The listing builds one solid part. Answer for the finished solid, in the listing's coordinates (mm). A direction names the side the tool comes from. Coordinates: 2 decimals unless noted, no trailing zeros. Order: outer loops, then holes, each group sorted by start corner. A loop starts at its lowest first (then second) coordinate and runs counter-clockwise, first axis right, second up. Notation, with made-up numbers: (-37, 49.25) - (-31, 49.25) arc R27 cw to (-31, 80.25) - close; hole circle Ø11 at (-28, 85.5). An arc over 180 degrees is marked (long way). Use one line per item in the form item = value. Start each with the question number.
Item 1: A tool of negligible diameter and unlimited length cuts with its end or side. For faces 1 (the flat face through (70, -93, -3)), 2 (the flat face through (78, -88, -4)), 3 (the flat face through (65.5, -96, -4)), from which of +Z, -Z, +X, -X, +Y, -Y can it reach the whole face along a straight path? Write none if from no direction.
Item 2: The mould has two halves that part along Y. Classify faces 4 (the flat face through (40, 2, 1)), 5 (the flat face through (78, -43, -4)), 6 (the flat face through (80.5, -58.4, 0.4)): released by +Y, released by -Y, zero draft, split by the parting line, or undercut.
Item 3: Consider line 1 along Y through (x, z) = (78.4, -4); line 2 along Z through (x, y) = (78, -38); line 3 along Y through (x, z) = (27, 1). Determine where each line is inside the solid, lowest interval first. Write a range as [from, to].
Item 4: Section C-C, the plane x = 19.5 is taken. Write down the section's boundary in (y, z).
Item 5: Section B-B, the plane y = -48 is taken. Write down the section's boundary in (x, z), and give its area (3 significant figures).
Item 6: Each of these flat-tipped pins is pushed along its axis until it touches: pin 1 Ø1 at (x, z) = (42.5, -6.5) entering from +Y; pin 2 Ø4 at (y, z) = (-90, -4) entering from -X; pin 3 Ø4 at (x, z) = (77, -5) entering from +Y; pin 4 Ø1.2 at (x, z) = (70.5, -4) entering from -Y. Where does it stop, or does it pass through?
Item 7: Section A-A, the plane y = -4 is taken. Write down the section's boundary in (x, z), and give its area (3 significant figures).
Item 8: Section D-D, the plane y = -18 is taken. Write down the section's boundary in (x, z), and give its area (3 significant figures).
Autodesk Inventor part; units mm, degrees
ref_plane "YZ Plane" through (0, 0, 0) normal (1, 0, 0) x (0, 1, 0)
ref_plane "XZ Plane" through (0, 0, 0) normal (0, 1, 0) x (-1, 0, 0)
ref_plane "XY Plane" through (0, 0, 0) normal (0, 0, 1) x (1, 0, 0)
ref_plane "Work Plane1" through (0, 0, 0) normal (0, 0, 1) x (1, 0, 0)
sketch "Sketch1" plane through (0, 0, 0) normal (0, 0, 1) x (1, 0, 0)
  line L0 (-2, -98) -> (8, -98)
  line L1 (-2, -98) -> (-2, 2)
  circle A0 centre (4, -93) radius 0.75
  circle A1 centre (4, -48) radius 0.75
  circle A2 centre (5, -4) radius 0.75
  line L2 (0, 2) -> (80.5, 2)
  circle A3 centre (40.25, -4) radius 0.75
  circle A4 centre (75.5, -4) radius 0.75
  line L3 (34.223, -24.7194) -> (34.223, -14.2194)
  line L4 (26.723, -24.7194) -> (34.223, -24.7194)
  line L5 (26.723, -14.2194) -> (26.723, -24.7194)
  line L6 (34.223, -14.2194) -> (26.723, -14.2194)
  line L7 (80.5, 2) -> (-2, 2)
  line L8 (-2, 2) -> (-2, -98)
  line L9 (-2, -98) -> (80.5, -98)
  line L10 (80.5, -98) -> (80.5, 2)
  point P0 (0, 0)
  point P1 (20.6901, -14.1894)
extrude "Extrusion1" add sketch "Sketch1" along normal blind 2
sketch "Sketch2" plane through (0, 0, 0) normal (0, 0, -1) x (-1, 0, 0)
  point P0 (0, 0)
sketch "Sketch3" plane through (0, 0, 0) normal (0, 0, -1) x (-1, 0, 0)
  point P0 (0, 0)
sketch "Sketch4" plane through (80.5, -98, 0) normal (1, 0, 0) x (0, 0, -1)
  line L0 (0, 45) -> (0, 55)
  line L1 (0, 45) -> (5, 45)
  line L2 (5, 55) -> (5, 45)
  line L3 (0, 55) -> (5, 55)
  line L4 (0, 45) -> (8, 45)
  line L5 (8, 45) -> (8, 55)
  line L6 (8, 55) -> (0, 55)
  circle A0 centre (4, 50) radius 0.75
  point P0 (0, 98)
  dimension "d3" = 8
  dimension "d4" = 10
  dimension "d6" = 1.5
extrude "Extrusion2" add sketch "Sketch4" against normal blind 5
sketch "Sketch5" plane through (80.5, -98, 2) normal (1, 0, 0) x (0, 0, -1)
  line L0 (2, 45) -> (2, 0)
  line L1 (2, 0) -> (10, 0)
  line L2 (10, 0) -> (10, 10)
  line L3 (10, 10) -> (2, 10)
  line L4 (2, 10) -> (2, 0)
  circle A0 centre (6, 5) radius 0.75
  point P0 (2, 98)
  dimension "d9" = 8
  dimension "d10" = 10
  dimension "d12" = 1.5
extrude "Extrusion3" add sketch "Sketch5" against normal blind 5
sketch "Sketch6" plane through (-2, -98, 2) normal (0, -1, 0) x (1, 0, 0)
  line L0 (77.5, -10) -> (77.5, -2)
  line L1 (77.5, -10) -> (67.5, -10)
  line L2 (67.5, -10) -> (67.5, -2)
  line L3 (67.5, -2) -> (77.5, -2)
  line L4 (77.5, -2) -> (77.5, -10)
  circle A0 centre (72.5, -6) radius 0.75
  point P0 (2, -2)
  dimension "d15" = 10
  dimension "d16" = 8
  dimension "d18" = 1.5
extrude "Extrusion4" add sketch "Sketch6" against normal blind 5
sketch "Sketch7" plane through (-2, -98, 2) normal (0, -1, 0) x (1, 0, 0)
  line L0 (10, -2) -> (10, -17)
  line L1 (67.5, -10) -> (67.5, -2)
  circle A0 centre (32.473, -6) radius 0.75
  line L2 (32.473, -10) -> (27.473, -10)
  line L3 (27.473, -10) -> (27.473, -2)
  line L4 (27.473, -2) -> (37.473, -2)
  line L5 (37.473, -2) -> (37.473, -10)
  line L6 (37.473, -10) -> (32.473, -10)
  point P0 (2, -2)
  dimension "d22" = 1.5
  dimension "d25" = 4
  dimension "d26" = 5
  dimension "d27" = 8
  dimension "d28" = 10
  dimension "d29" = 8
extrude "Extrusion5" add sketch "Sketch7" against normal blind 5
sketch "Sketch8" plane through (-2, -98, 2) normal (0, -1, 0) x (1, 0, 0)
  line L0 (37.473, -10) -> (27.473, -10)
  line L1 (27.473, -10) -> (37.473, -10)
  line L2 (37.473, -10) -> (37.473, -2)
  line L3 (37.473, -2) -> (27.473, -2)
  line L4 (27.473, -2) -> (27.473, -10)
  point P0 (2, -2)
extrude "Extrusion6" cut sketch "Sketch8" against normal blind 5
sketch "Sketch9" plane through (-2, -98, 2) normal (0, -1, 0) x (1, 0, 0)
  line L0 (47.25, -2) -> (47.25, -7)
  line L1 (47.25, -7) -> (37.25, -7)
  line L2 (37.25, -7) -> (37.25, -2)
  line L3 (37.25, -2) -> (47.25, -2)
  line L4 (67.5, -2) -> (0, -2)
  line L5 (37.25, -2) -> (37.25, -10)
  line L6 (37.25, -10) -> (47.25, -10)
  line L7 (47.25, -10) -> (47.25, -2)
  line L8 (47.25, -2) -> (37.25, -2)
  circle A0 centre (42.25, -6) radius 0.75
  point P0 (2, -2)
  dimension "d35" = 8
  dimension "d36" = 10
  dimension "d38" = 1.5
extrude "Extrusion7" add sketch "Sketch9" against normal blind 5
sketch "Sketch10" plane through (80.5, -53, -8) normal (0, 0, -1) x (-1, 0, 0)
  line L0 (5, 10) -> (5, 0)
  line L1 (0, -45) -> (0, 55)
  line L2 (5, 0) -> (0, 0)
  line L3 (0, 0) -> (0, 10)
  line L4 (0, 10) -> (5, 10)
  line L5 (5, 10) -> (5, 0)
  point P0 (80.5, 53)
  dimension "d41" = 10
extrude "Extrusion8" cut sketch "Sketch10" against normal blind 8
sketch "Sketch11" plane through (0, 0, 0) normal (0, 0, -1) x (-1, 0, 0)
  circle A0 centre (-4, -48) radius 0.75
  line L0 (-80.5, 2) -> (-80.5, -88)
  line L1 (-80.5, -48) -> (-80.5, -43)
  line L2 (-80.5, -43) -> (-80.5, -33)
  line L3 (-80.5, -33) -> (-75.5, -33)
  line L4 (-75.5, -33) -> (-75.5, -43)
  line L5 (-75.5, -43) -> (-80.5, -43)
  point P0 (0, 0)
  dimension "d44" = 5
  dimension "d45" = 10
  dimension "d46" = 5
  dimension "d47" = 10
extrude "Extrusion9" add sketch "Sketch11" along normal blind 8 contours L3 L4 L5 L0
sketch "Sketch12" plane through (80.5, -98, 2) normal (1, 0, 0) x (0, 0, -1)
  line L0 (10, 65) -> (10, 55)
  circle A0 centre (6, 60) radius 0.75
  point P0 (2, 98)
  dimension "d51" = 1.5
extrude "Extrusion10" cut sketch "Sketch12" against normal blind 5
sketch "Sketch13" plane through (0, 0, 2) normal (0, 0, 1) x (1, 0, 0)
  circle A0 centre (5, -4) radius 0.75
  circle A1 centre (5, -4) radius 1.25
  circle A2 centre (40.25, -4) radius 0.75
  circle A3 centre (40.25, -4) radius 1.25
  circle A4 centre (75.5, -4) radius 0.75
  circle A5 centre (75.5, -4) radius 1.25
  circle A6 centre (4, -48) radius 0.75
  circle A7 centre (4, -48) radius 1.25
  circle A8 centre (4, -93) radius 0.75
  circle A9 centre (4, -93) radius 1.25
  point P0 (0, 0)
  dimension "d54" = 2.5
  dimension "d55" = 2.5
  dimension "d56" = 2.5
  dimension "d57" = 2.5
  dimension "d58" = 2.5
extrude "Extrusion11" cut sketch "Sketch13" against normal blind 2
properties part number "Lateral Derecho" material "Nylon 6/6"
Response:
q1.face_1 = -Z, -X, +Y
q1.face_2 = -Z, +X, -X
q1.face_3 = -Z, +Y, -Y
q2.face_4 = released by +Y
q2.face_5 = undercut
q2.face_6 = zero draft
q3.line_1 = [-98, -93.75], [-92.25, -88], [-43, -38.75], [-37.25, -33]
q3.line_2 = [-8, -4.75], [-3.25, 2]
q3.line_3 = [-98, -24.72], [-14.22, 2]
q4.outline = (-98, 0) - (2, 0) - (2, 2) - (-98, 2) - close
q5.outline = (-2, 0) - (2.75, 0) - (2.75, 2) - (-2, 2) - close; (5.25, 0) - (80.5, 0) - (80.5, 2) - (5.25, 2) - close
q5.area = 160 mm2
q6.pin_1 = -93
q6.pin_2 = 75.5
q6.pin_3 = -33
q6.pin_4 = through
q7.outline = (-2, 0) - (3.75, 0) - (3.75, 2) - (-2, 2) - close; (6.25, 0) - (39, 0) - (39, 2) - (6.25, 2) - close; (41.5, 0) - (74.25, 0) - (74.25, 2) - (41.5, 2) - close; (76.75, 0) - (80.5, 0) - (80.5, 2) - (76.75, 2) - close
q7.area = 150 mm2
q8.outline = (-2, 0) - (26.72, 0) - (26.72, 2) - (-2, 2) - close; (34.22, 0) - (80.5, 0) - (80.5, 2) - (34.22, 2) - close
q8.area = 150 mm2
